```python
from build123d import *

# Parameters (mm, degrees)
F0_R     = 3.176712
F0_W     = 60.944215
F0_H     = 25.435724
F0_R_2   = 3.170316
F0_R_3   = 4.447947
F0_R_4   = 3.175147
F0_W_2   = 60.941307
F0_R_5   = 3.171767
F1_DEPTH = 7.62


with BuildPart() as f1:
    # F0 (on Top) → F1 (new body)
    with BuildSketch(Plane.XY):
        Polygon((0, -10.154884), (0, 0), (-10.158613, 0), (-15.246199, 0), (-44.828615, 0), (-76.187506, 0), (-86.349189, 0), (-86.349189, -10.154884), (-93.980744, -10.154884), (-93.980744, 0), (-104.15256, 0), (-165.096775, 0), (-170.221075, 0), (-180.353627, 0), (-180.353627, -10.154884), (-180.353627, -35.590608), (-180.353627, -45.754101), (-170.221075, -45.754101), (-165.096775, -45.754101), (-93.980744, -45.754101), (-93.980744, -35.590608), (-86.349189, -35.590608), (-86.349189, -45.754101), (-76.187506, -45.754101), (-15.246199, -45.754101), (-10.158613, -45.754101), (0, -45.754101), (0, -35.590608), align=None)
        with Locations((-172.680676, -22.530714)):
            Circle(F0_R, mode=Mode.SUBTRACT)
        with Locations((-134.624667, -22.872746)):
            Rectangle(F0_W, F0_H, mode=Mode.SUBTRACT)
        with Locations((-99.302329, -22.530714)):
            Circle(F0_R_2, mode=Mode.SUBTRACT)
        with Locations((-90.164967, -22.530714)):
            Circle(F0_R_3, mode=Mode.SUBTRACT)
        with Locations((-80.425173, -22.530714)):
            Circle(F0_R_4, mode=Mode.SUBTRACT)
        with Locations((-45.716853, -22.872746)):
            Rectangle(F0_W_2, F0_H, mode=Mode.SUBTRACT)
        with Locations((-7.969475, -22.877051)):
            Circle(F0_R_5, mode=Mode.SUBTRACT)
    extrude(amount=F1_DEPTH)


solid = f1.part
```
For this review, take the finished solid that the model builds, in its own axes (mm). A direction names the side the tool comes from. Coordinates: 2 decimals unless noted, no trailing zeros. Loops run counter-clockwise (first coordinate to the right, second up) from the corner with the lowest first, then second, coordinate; pieces in that order, holes last. Notation, with made-up numbers: (76.5, -36.5) -> (103.5, -36.5) arc R13 ccw to (103.5, -29.5) -> close; hole circle Ø8 at (68, -18). An arc over 180 degrees is marked (long way). Return JSON: item names as keys, results as strings. Group by question number.
(1) Consider section A-A, the plane x = -111. Give the boundary of the cut face in (y, z).
(2) For pin 1 Ø4 at (x, z) = (-89, 3.5) entering from -Y, flat-tipped, find the tip position at first contact; note if it passes through.
(3) Consider section C-C, the plane z = 2.75. Give the boundary of the cut face in (x, y).
(4) Tool access review of faces 4 (the flat face through (-93.981, -5, 4)), 5 (the flat face through (-90, -35.591, 4)), 6 (the flat face through (-137, 0, 4)), 7 (the flat face through (-91, -17, 7.62)), 8 (the flat face through (-135, -35.591, 4)): name each direction out of +Z, -Z, +X, -X, +Y, -Y from which nothing blocks a thin tool from reaching the whole face with its end or side.
(5) Consider section B-B, the plane y = -42. Give the boundary of the cut face in (x, z), plus the area to 3 significant figures.
(6) Mouldability with a two-part tool opening along X and no side actions: class faces 1 (the flat face through (-43, 0, 4)), 2 (the flat face through (0, -23, 4)), 3 (the flat face through (-165.097, -23, 4)) as pulls with the +X half, pulls with the -X half, needs draft (parallel to the pull), parting line crosses it, or undercut.
(7) To check wall thickness, follow L1, parallel to X at y = -30.5, z = 5.5; L2, parallel to Y at x = -27.5, z = 1.5; L3, parallel to X at y = -42.5, z = 6.5. State the ranges of each line that lie inside material, in increasing order.
Results below:
{
 "1": {"outline": "(-45.75, 0) -> (-35.59, 0) -> (-35.59, 7.62) -> (-45.75, 7.62) -> close; (-10.15, 0) -> (0, 0) -> (0, 7.62) -> (-10.15, 7.62) -> close"},
 "2": {"pin 1": "stops at y = -35.59"},
 "3": {"outline": "(-180.35, -45.75) -> (-93.98, -45.75) -> (-93.98, -35.59) -> (-86.35, -35.59) -> (-86.35, -45.75) -> (0, -45.75) -> (0, 0) -> (-86.35, 0) -> (-86.35, -10.15) -> (-93.98, -10.15) -> (-93.98, 0) -> (-180.35, 0) -> close; hole circle Ø6.35 at (-172.68, -22.53); hole (-165.1, -35.59) -> (-104.15, -35.59) -> (-104.15, -10.15) -> (-165.1, -10.15) -> close; hole circle Ø6.34 at (-99.3, -22.53); hole circle Ø8.9 at (-90.16, -22.53); hole circle Ø6.35 at (-80.43, -22.53); hole (-76.19, -35.59) -> (-15.25, -35.59) -> (-15.25, -10.15) -> (-76.19, -10.15) -> close; hole circle Ø6.34 at (-7.97, -22.88)"},
 "4": {"face 4": "+Z, -Z, +Y", "face 5": "+Z, -Z, -Y", "face 6": "+Z, -Z, +X, -X, +Y", "face 7": "+Z, +X, -X, +Y, -Y", "face 8": "+Z, -Z"},
 "5": {"outline": "(-180.35, 0) -> (-93.98, 0) -> (-93.98, 7.62) -> (-180.35, 7.62) -> close; (-86.35, 0) -> (0, 0) -> (0, 7.62) -> (-86.35, 7.62) -> close", "area": "1,320 mm2"},
 "6": {"face 1": "needs draft", "face 2": "pulls with the +X half", "face 3": "undercut"},
 "7": {"L1": "x = -180.35 to -165.1, -104.15 to -76.19, -15.25 to 0", "L2": "y = -45.75 to -35.59, -10.15 to 0", "L3": "x = -180.35 to -93.98, -86.35 to 0"}
}
